For this review, use the dimensioned drawing (mm, ordinates from the lowest corner) and the shaded views. Give positions to 0.01 mm unless a question says otherwise; leave off trailing zeros. Loops run counter-clockwise (first coordinate to the right, second up) from the corner with the lowest first, then second, coordinate; pieces in that order, holes last. Notation, with made-up numbers: M 88.5,38 L 128.5,38 A17 cw 128.5,53 Z; hole C 13,2 d1. An arc over 180 degrees is marked long. Return JSON: item names as keys, results as strings.
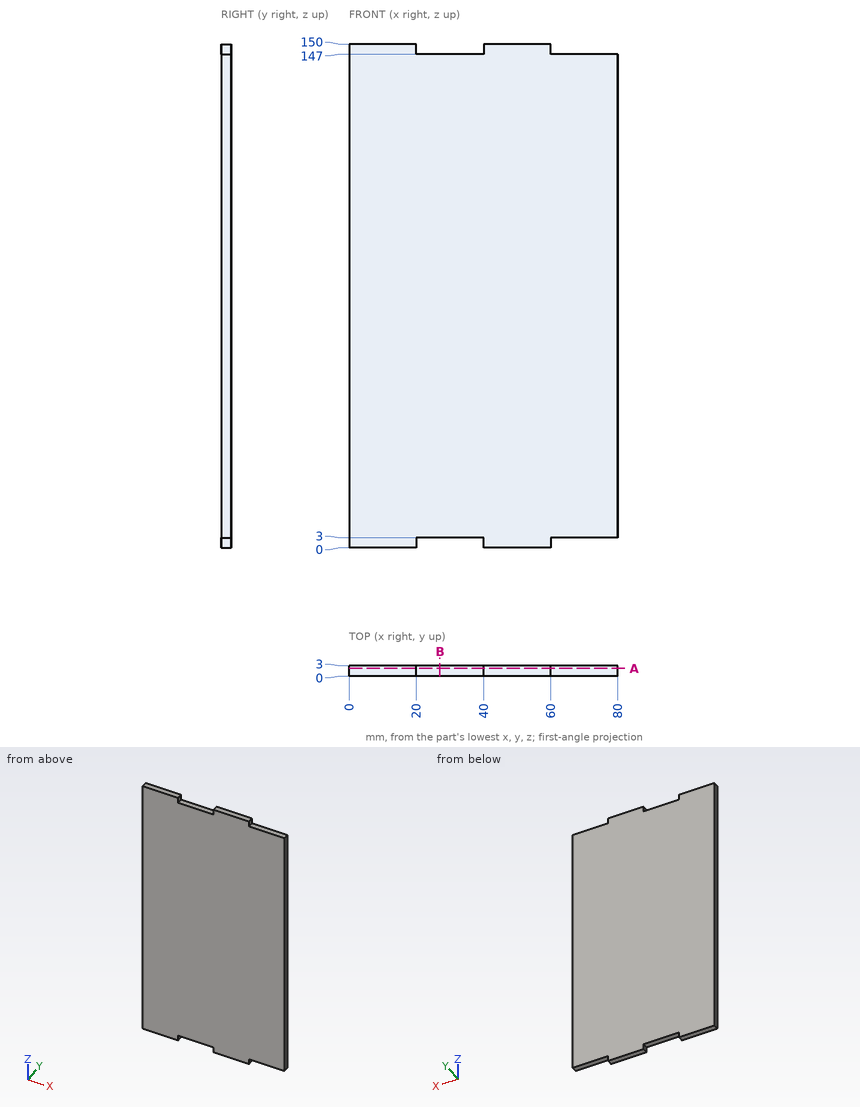
1) Consider section A-A on y = 2.3. Write out the cut boundary in (x, z).
From the geometry:
{"outline": "M 0,0 L 20,0 L 20,3 L 40,3 L 40,0 L 60,0 L 60,3 L 80,3 L 80,147 L 60,147 L 60,150 L 40,150 L 40,147 L 20,147 L 20,150 L 0,150 Z"}
2) Wall thickness on L1, parallel to Z at x = 65, y = 0.9: over which ranges is the line inside the solid? List them lowest first. Write a range as from..to.
From the geometry:
{"L1": "3..147"}
3) Insertion check: pin 1 (1.5 mm diameter, centred on y = 1.5, z = 148.5, fed in from +X); pin 2 (1.5 mm diameter, centred on x = 28, y = 2, fed in from -Z). Each pin has a flat end and moves straight along its axis. Give the tip position at first contact, or say it passes through.
From the geometry:
{"pin 1": "x = 60", "pin 2": "z = 3"}
4) Consider section B-B on x = 27. Write out the cut boundary in (y, z), then the cut area to 3 significant figures.
From the geometry:
{"outline": "M 0,3 L 3,3 L 3,147 L 0,147 Z", "area": "432 mm²"}
